Here's how the part is built. I have some questions about the finished solid (model axes, mm). Face numbers are marked on the shaded views. A direction names the side the tool comes from. Give positions to 0.01 mm unless a question says otherwise; leave off trailing zeros. Order: outer loops, then holes, each group sorted by start corner. A loop starts at its lowest first (then second) coordinate and runs counter-clockwise, first axis right, second up. Notation, with made-up numbers: (36.25, 66.25) -> (79.25, 66.25) arc R18 cw to (79.25, 79.25) -> close; hole circle Ø7 at (52, 33.25). An arc over 180 degrees is marked (long way). Write each question's results on one line, items separated by ' | '. Start each with the question number.
Q1. For the marked faces 1 and 2, which set-ups out of +Z, -Z, +X, -X, +Y, -Y let a thin tool reach every point of the face, with its end or its side?
Q2. I'm going to push flat-ended pins straight in: pin 1 (14.5 mm diameter, centred on x = -54.99, z = -31.75, fed in from +Y); pin 2 (3 mm diameter, centred on y = 41, z = 36, fed in from +X); pin 3 (12 mm diameter, centred on x = -10, z = -17, fed in from -Y); pin 4 (11.5 mm diameter, centred on x = 0, z = 63.5, fed in from -Y). Where does each tip first touch, or does it pass through?
Q3. Imagine slicing it at B-B, the plane y = 5. Please give me the cut outline in (x, z), then the cut area to 3 significant figures.
Q4. Imagine slicing it at A-A, the plane x = 0. State how many separate pieces and enclosed holes the cut face has, then the cut area to 3 significant figures.
Q5. I need wall thicknesses on line 1 along X through (y, z) = (-39, 31); line 2 along X through (y, z) = (25, 0); line 3 along X through (y, z) = (-18.75, 0). Which ranges of each line are inside material? Lowest first, please. Write a range as [from, to].
Q6. Thinking about a two-plate mould opening in Z: for the marked faces 3, 4, 5 and 6, which applies, pulls with the +Z half, pulls with the -Z half, needs draft (parallel to the pull), parting line crosses it, or undercut?
```python
from build123d import *

# Parameters (mm, degrees)
F3_SIZE  = 1.905
F4_R     = 5.08
F5_R     = 6.35
F6_DEPTH = 15.875


with BuildPart() as f1:
    # F0 (on Right) → F1 (revolve)
    with BuildSketch(Plane.YZ):
        Polygon((-44.526481, 38.1), (-44.526481, 25.4), (-25.476481, 25.4), (-25.476481, 28.860142), (-12.776481, 28.860142), (-12.776481, 25.4), (57.073519, 25.4), (57.073519, 38.1), (-7.818043, 38.1), (-7.818043, 50.8), (-33.218043, 50.8), (-33.218043, 76.2), (-44.526481, 76.2), align=None)
    revolve(axis=Axis((0, 16.093373, 0), (0, 1, 0)))

    # F3
    f3_edges = [f1.edges().sort_by_distance(p)[0] for p in [
        (0, -44.526481, -76.2),
        (0, -33.218043, -76.2),
        (0, -7.818043, -50.8),
        (0, 57.073519, -38.1),
        (0, -44.526481, -25.4),
    ]]
    chamfer(f3_edges, length=F3_SIZE)

    # F4
    f4_edges = [f1.edges().sort_by_distance(p)[0] for p in [
        (0, -33.218043, -50.8),
        (0, -7.818043, -38.1),
    ]]
    fillet(f4_edges, radius=F4_R)

    # F5 (on face) → F6 (cut)
    with BuildSketch(Plane.XZ.offset(44.526481)):
        with Locations((-54.992613, 31.75)):
            Circle(F5_R)
        with Locations((-54.992613, -31.75)):
            Circle(F5_R)
        with Locations((0, -63.5)):
            Circle(F5_R)
        with Locations((54.992613, -31.75)):
            Circle(F5_R)
        with Locations((54.992613, 31.75)):
            Circle(F5_R)
        with Locations((0, 63.5)):
            Circle(F5_R)
    extrude(amount=-F6_DEPTH, mode=Mode.SUBTRACT)


solid = f1.part
```
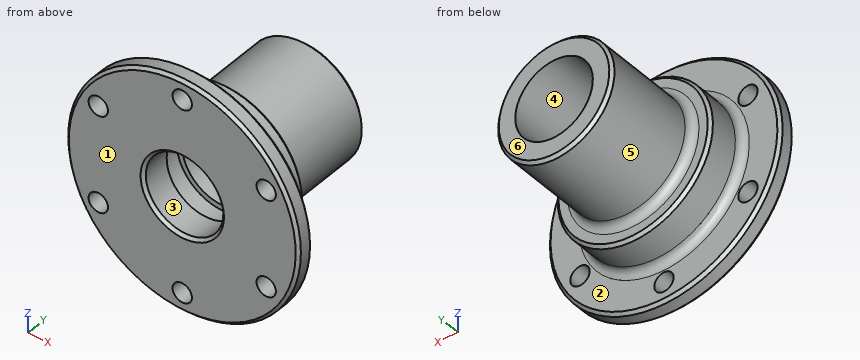
Geometry check:
1) face 1: +Z, -Z, +X, -X, -Y | face 2: +Y
2) pin 1: y = -33.22 | pin 2: x = 16.17 | pin 3: y = -42.94 | pin 4: through
3) outline: circle Ø76.2 at (0, 0); hole circle Ø50.8 at (0, 0) | area: 2,530 mm²
4) separate pieces: 4 | enclosed holes: 0 | area: 3,720 mm²
5) line 1: [-69.61, -61.3], [-48.69, 48.69], [61.3, 69.61] | line 2: [-38.1, -25.4], [25.4, 38.1] | line 3: [-50.8, -28.86], [28.86, 50.8]
6) face 3: undercut | face 4: undercut | face 5: parting line crosses it | face 6: needs draft
